For this review, use the dimensioned drawing (mm, ordinates from the lowest corner) and the shaded views. A direction names the side the tool comes from. Give positions to 0.01 mm unless a question says otherwise; leave off trailing zeros. Write each loop counter-clockwise with the first axis right and the second up, starting at its lowest first coordinate (ties: lowest second). Pieces come first, ordered by that corner, then holes.
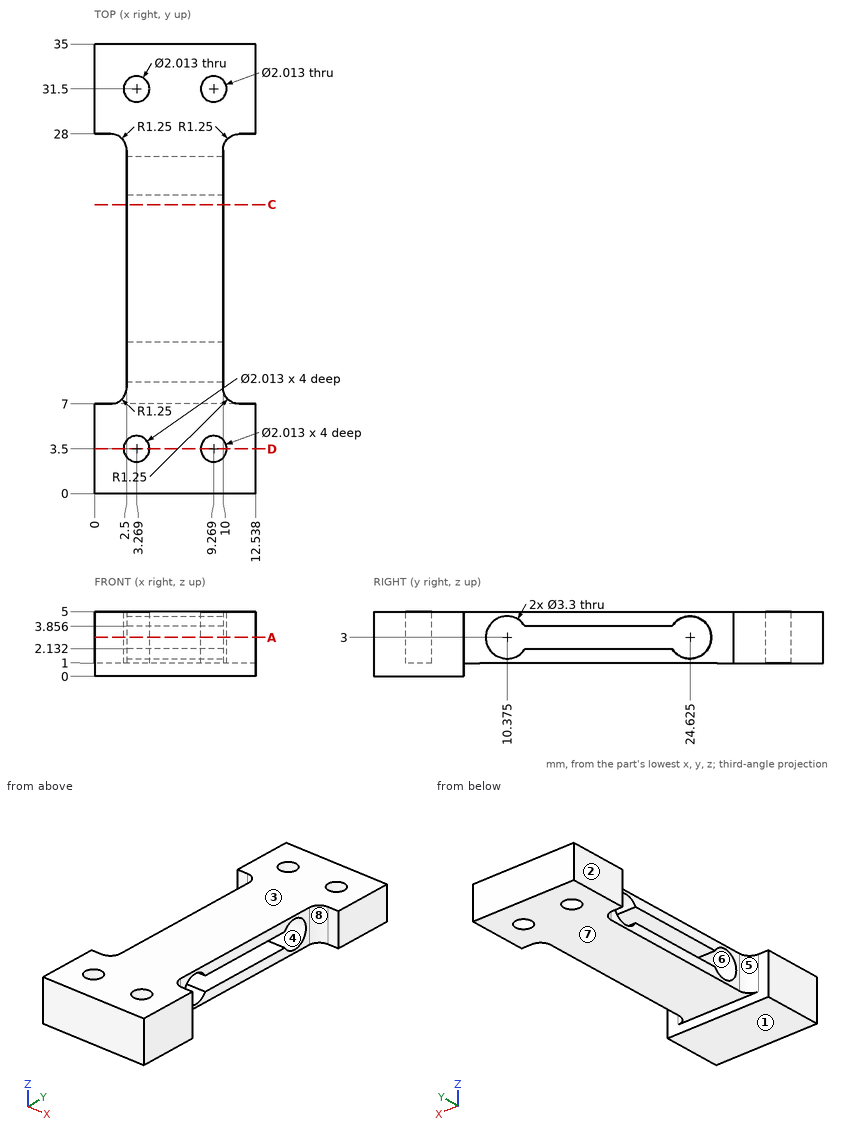
(1) We need section A-A (z = 3). Count the separate pieces of the cut face and the enclosed holes in it, and give its area (3 significant figures).
(2) Clearance check with flat-ended pins moving along their axes: pin 1 Ø1.5 at (y, z) = (22.5, 1.5) entering from -X; pin 2 Ø1 at (x, y) = (11, 18) entering from +Z; pin 3 Ø1 at (x, y) = (3.5, 3.5) entering from +Z; pin 4 Ø3 at (y, z) = (14, 2) entering from +X. State where each tip first meets the part, or that it passes through.
(3) We need section D-D (y = 3.5). Write out the cut boundary in (x, z) (1 decimal).
(4) For L1, parallel to Y at x = 4, z = 2.6 (1 decimal); L2, parallel to Z at x = 5.5, y = 14; L3, parallel to Y at x = 0.75, z = 3.3, list the stretches that pass through material, from the lowest coordinate up.
(5) Tool access review of the marked faces 5, 6, 7 and 8: name each direction out of +Z, -Z, +X, -X, +Y, -Y from which nothing blocks a thin tool from reaching the whole face with its end or side.
(6) The part is to be moulded in two halves that separate along Z. For the marked faces 1, 2, 3 and 4, say which applies: +Z half, -Z half, draft (parallel to the pull), parting line (faces both ways), or undercut.
(7) We need section C-C (y = 22.5). Write out the cut boundary in (x, z).
The answers:
1. separate pieces: 2
1. enclosed holes: 4
1. area: 190 mm2
2. pin 1: stops at x = 2.5
2. pin 2: passes through
2. pin 3: stops at z = 1
2. pin 4: stops at x = 10
3. outline: (0, 0) - (12.5, 0) - (12.5, 5) - (10.3, 5) - (10.3, 1) - (8.3, 1) - (8.3, 5) - (4.3, 5) - (4.3, 1) - (2.3, 1) - (2.3, 5) - (0, 5) - close
4. L1: y = 0 to 2.8, 4.2 to 8.8, 26.2 to 30.8, 32.2 to 35
4. L2: z = 1 to 2.13, 3.86 to 5
4. L3: y = 0 to 7, 28 to 35
5. face 5: +Z, -Z, -X
5. face 6: +X, -X
5. face 7: -Z, +X, -X, +Y
5. face 8: +Z, -Z, +X
6. face 1: -Z half
6. face 2: draft
6. face 3: +Z half
6. face 4: undercut
7. outline: (2.5, 1) - (10, 1) - (10, 2.13) - (2.5, 2.13) - close; (2.5, 3.86) - (10, 3.86) - (10, 5) - (2.5, 5) - close
